Source: CAD feature listing. Evaluate the final solid. Frame: model axes, mm. A direction names the side the tool comes from. Round coordinates to 2 decimals unless told otherwise and drop trailing zeros. Order: outer loops, then holes, each group sorted by start corner. A loop starts at its lowest first (then second) coordinate and runs counter-clockwise, first axis right, second up. Notation, with made-up numbers: (77, 69) -> (135, 69) arc R30 cw to (135, 97) -> close; hole circle Ø6 at (-12, 86). An arc over 180 degrees is marked (long way). Answer as CSV lines item,"result".
from build123d import *

# Parameters (mm, degrees)
BOSS_EXTRUDE2_DEPTH    = 127
CONVERT_SOLID1_START   = -127
CONVERT_SOLID1_DEPTH   = 254
CONVERT_SOLID1_2_DEPTH = 254
SKETCH7_R              = 6.35
SKETCH7_R_2            = 3.175
CUT_EXTRUDE1_DEPTH     = 513.718362651
SKETCH8_R              = 3.175
CUT_EXTRUDE2_DEPTH     = 25.4
BOSS_EXTRUDE3_DEPTH    = 3.175
SKETCH10_R             = 6.35
SKETCH10_R_2           = 1.25
CUT_EXTRUDE3_DEPTH     = 3.175
HEM1_START             = -238.125
HEM1_DEPTH             = 476.25


# Read off the part's stored shape, not the designer's step: Convert-Solid1, Hem1
with BuildPart() as part:
    # Sketch1 → Boss-Extrude2 (new, symmetric)
    with BuildSketch(Plane(origin=(0, 0, 0), x_dir=(1, 0, 0), z_dir=(0, 1, 0))):
        Polygon((-244.475, 84.455), (-241.3, 84.455), (-241.3, -84.455), (241.3, -84.455), (241.3, 84.455), (244.475, 87.63), (244.475, -87.63), (-244.475, -87.63), align=None)
    extrude(amount=BOSS_EXTRUDE2_DEPTH, both=True)

    # Convert-Solid1 outline → Convert-Solid1 (cut)
    with BuildSketch(Plane(origin=(0, 0, 0), x_dir=(1, 0, 0), z_dir=(0, 1, 0)).offset(CONVERT_SOLID1_START)):
        Polygon((244.475, 87.63), (241.3, 84.455), (244.475, 84.455), align=None)
        with BuildLine():
            Line((-244.475, -87.63), (-238.125, -87.63))
            ThreePointArc((-238.125, -87.63), (-242.615128061, -85.770128061), (-244.475, -81.28))
            Line((-244.475, -81.28), (-244.475, -87.63))
        make_face()
        with BuildLine():
            Line((244.475, -87.63), (244.475, -81.28))
            ThreePointArc((244.475, -81.28), (242.615128061, -85.770128061), (238.125, -87.63))
            Line((238.125, -87.63), (244.475, -87.63))
        make_face()
    extrude(amount=CONVERT_SOLID1_DEPTH, mode=Mode.SUBTRACT)

    # Convert-Solid1 2 outline → Convert-Solid1 2 (add)
    with BuildSketch(Plane(origin=(0, 0, 0), x_dir=(1, 0, 0), z_dir=(0, 1, 0)).offset(CONVERT_SOLID1_START)):
        with BuildLine():
            Line((-241.3, -84.455), (-238.125, -84.455))
            ThreePointArc((-238.125, -84.455), (-240.37006403, -83.52506403), (-241.3, -81.28))
            Line((-241.3, -81.28), (-241.3, -84.455))
        make_face()
        with BuildLine():
            Line((241.3, -84.455), (241.3, -81.28))
            ThreePointArc((241.3, -81.28), (240.37006403, -83.52506403), (238.125, -84.455))
            Line((238.125, -84.455), (241.3, -84.455))
        make_face()
    extrude(amount=CONVERT_SOLID1_2_DEPTH)

    # Sketch7 → Cut-Extrude1 (cut, through all)
    with BuildSketch(Plane.ZY.offset(244.475)):
        with Locations((-57.15, 155.575)):
            Circle(SKETCH7_R)
        with Locations((-57.15, 104.14)):
            Circle(SKETCH7_R)
        with Locations((-57.15, 52.705)):
            Circle(SKETCH7_R)
        with Locations((-57.15, 1.27)):
            Circle(SKETCH7_R)
        with Locations((-57.15, -50.165)):
            Circle(SKETCH7_R)
        with Locations((-57.15, 207.01)):
            Circle(SKETCH7_R)
        with Locations((-57.15, -101.6)):
            Circle(SKETCH7_R)
        with Locations((-44.45, -24.4475)):
            Circle(SKETCH7_R_2)
        with Locations((-44.45, 26.9875)):
            Circle(SKETCH7_R_2)
        with Locations((-44.45, -75.8825)):
            Circle(SKETCH7_R_2)
    extrude(amount=-CUT_EXTRUDE1_DEPTH, mode=Mode.SUBTRACT)

    # Sketch8 → Cut-Extrude2 (cut)
    with BuildSketch(Plane.XY.offset(87.63)):
        with Locations((0, 114.3)):
            Circle(SKETCH8_R)
        with Locations((228.6, 114.3)):
            Circle(SKETCH8_R)
        with Locations((-228.6, 114.3)):
            Circle(SKETCH8_R)
    extrude(amount=-CUT_EXTRUDE2_DEPTH, mode=Mode.SUBTRACT)

    # Sketch9 → Boss-Extrude3 (add)
    with BuildSketch(Plane.ZY.offset(244.475)):
        with BuildLine():
            Line((-84.455, -46.344167394), (-116.205, -64.675038441))
            ThreePointArc((-116.205, -64.675038441), (-128.905, -86.672083697), (-116.205, -108.669128953))
            Line((-116.205, -108.669128953), (-84.455, -127))
            Line((-84.455, -127), (-84.455, -46.344167394))
        make_face()
    extrude(amount=-BOSS_EXTRUDE3_DEPTH)

    # Sketch10 → Cut-Extrude3 (cut)
    with BuildSketch(Plane.ZY.offset(244.475)):
        with Locations((-96.505, -86.672083697)):
            Circle(SKETCH10_R)
        with Locations((-90.081606241, -94.422083697)):
            Circle(SKETCH10_R_2)
        with Locations((-116.928393759, -94.422083697)):
            Circle(SKETCH10_R_2)
        with Locations((-116.928393759, -78.922083697)):
            Circle(SKETCH10_R_2)
        with Locations((-90.081606241, -78.922083697)):
            Circle(SKETCH10_R_2)
    extrude(amount=-CUT_EXTRUDE3_DEPTH, mode=Mode.SUBTRACT)

    # Hem1 outline → Hem1 (add)
    with BuildSketch(Plane.YZ.offset(HEM1_START)):
        with BuildLine():
            Line((-230.183232322, 1.048987815), (-227.056467706, 0.497654851))
            ThreePointArc((-227.056467706, 0.497654851), (-192.307221144, 60.685115421), (-127, 84.455))
            Line((-127, 84.455), (-127, 87.63))
            ThreePointArc((-127, 87.63), (-194.348071805, 63.117306528), (-230.183232322, 1.048987815))
        make_face()
    extrude(amount=HEM1_DEPTH)


solid = part.part
1. Section query D-D on x = -139. Return loops of the section in (y, z) (3 decimals).
Results below:
outline,"(-230.183, 1.049) -> (-227.056, 0.498) arc R101.6 cw to (-127, 84.455) -> (127, 84.455) -> (127, 87.63) -> (-127, 87.63) arc R104.775 ccw to start"
2. Section query B-B on z = -5. Return loops of the section in (x, y) (3 decimals).
Results below:
outline,"(-244.475, -127) -> (-241.3, -127) -> (-241.3, 127) -> (-244.475, 127) -> close; (241.3, -127) -> (244.475, -127) -> (244.475, 127) -> (241.3, 127) -> close"
3. Mould query, pull axis X, two halves, no side actions, for faces 3 (the flat face through (244.475, 2, -3)), 4 (the cylindrical face through (242.87, 48.84, -62.19)), 5 (the flat face through (-244.475, 2, -2)), 6 (the flat face through (-3, 2, 84.455)). Classes: released by +X, released by -X, zero draft, split by the parting line, or undercut.
Results below:
face 3,"released by +X"
face 4,"zero draft"
face 5,"released by -X"
face 6,"undercut"
4. Line query: L1, parallel to Y at x = -242.45, z = -57.15 (3 decimals); L2, parallel to Y at x = -242.25, z = -44.45; L3, parallel to X at y = 114, z = 86. Output: solid intervals per line, ascending. Write a range as [from, to].
Results below:
L1,"[-127, -107.95], [-95.25, -56.515], [-43.815, -5.08], [7.62, 46.355], [59.055, 97.79], [110.49, 127]"
L2,"[-127, -79.06], [-72.71, -27.62], [-21.27, 23.81], [30.16, 127]"
L3,"[-242.37, -231.76], [-225.44, -3.16], [3.16, 225.44], [231.76, 242.37]"
5. Section query C-C on z = 60. Return loops of the section in (x, y) (3 decimals), and give its area (3 significant figures).
Results below:
outline,"(-244.475, -127) -> (-241.3, -127) -> (-241.3, 127) -> (-244.475, 127) -> close; (-238.125, -197.897) -> (238.125, -197.897) -> (238.125, -193.115) -> (-238.125, -193.115) -> close; (241.3, -127) -> (244.475, -127) -> (244.475, 127) -> (241.3, 127) -> close"
area,"3,890 mm2"
6. Reachability of faces 1 (the flat face through (241.3, 2, 0)), 2 (the cylindrical face through (-242.91, -2.59, -62.19)) from +Z, -Z, +X, -X, +Y, -Y: full face, straight path, thin tool, end or side. Return the list, or none.
Results below:
face 1,"-Z, +Y, -Y"
face 2,"+X, -X"
7. Pin query (flat end, axial travel): pin 1 (7 mm diameter, centred on x = -240.5, z = 31.5, fed in from -Y); pin 2 (3.5 mm diameter, centred on x = -242.5, y = 65.5, fed in from -Z) (3 decimals); pin 3 (8 mm diameter, centred on x = -74, y = -53.5, fed in from -Z) (3 decimals). Return the tip coordinate at first contact, or that it passes through.
Results below:
pin 1,"y = -221.1"
pin 2,"z = -84.455"
pin 3,"z = 84.455"
8. Section query A-A on y = 104.14. Return loops of the section in (x, z) (3 decimals), and give its area (3 significant figures).
Results below:
outline,"(-244.475, -84.455) -> (-241.3, -84.455) -> (-241.3, -63.5) -> (-244.475, -63.5) -> close; (-244.475, -50.8) -> (-241.3, -50.8) -> (-241.3, 81.28) arc R3.175 cw to (-238.125, 84.455) -> (238.125, 84.455) arc R3.175 cw to (241.3, 81.28) -> (241.3, -50.8) -> (244.475, -50.8) -> (244.475, 81.28) arc R6.35 ccw to (238.125, 87.63) -> (-238.125, 87.63) arc R6.35 ccw to (-244.475, 81.28) -> close; (241.3, -84.455) -> (244.475, -84.455) -> (244.475, -63.5) -> (241.3, -63.5) -> close"
area,"2,530 mm2"
